Model file for the job. Use its own axes, mm. Face numbers are marked on the shaded views. Coordinates: 2 decimals unless noted, no trailing zeros. Order: outer loops, then holes, each group sorted by start corner. A loop starts at its lowest first (then second) coordinate and runs counter-clockwise, first axis right, second up. Notation, with made-up numbers: M 70,27 L 101,27 A25 ccw 101,58 Z; hole C -14,5.25 d4. An arc over 180 degrees is marked long. Return JSON: item names as keys, results as strings.
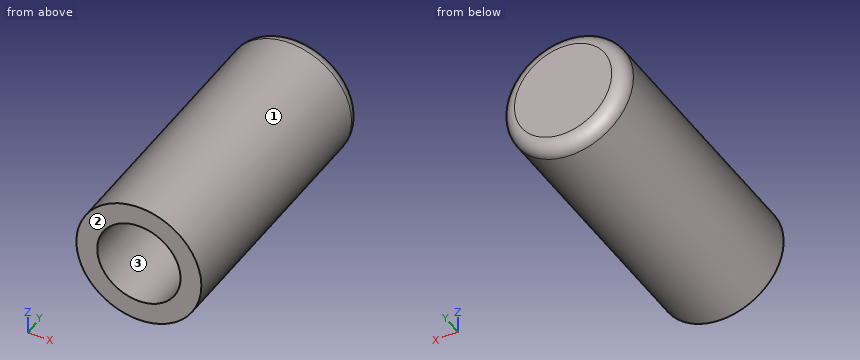
```python
from build123d import *

# Parameters (mm, degrees)
SKETCH2_R           = 4.5
SKETCH2_R_2         = 3
BOSS_EXTRUDE1_DEPTH = 20
SKETCH2_2_R         = 3
BOSS_EXTRUDE2_DEPTH = 2
FILLET1_R           = 1


with BuildPart() as part:
    # Sketch2 → Boss-Extrude1 (new body)
    with BuildSketch(Plane(origin=(0, 0, 0), x_dir=(1, 0, 0), z_dir=(0, 1, 0))):
        Circle(SKETCH2_R)
        Circle(SKETCH2_R_2, mode=Mode.SUBTRACT)
    extrude(amount=-BOSS_EXTRUDE1_DEPTH)

    # Sketch2<2> → Boss-Extrude2 (add)
    with BuildSketch(Plane(origin=(0, 0, 0), x_dir=(1, 0, 0), z_dir=(0, 1, 0))):
        Circle(SKETCH2_2_R)
    extrude(amount=-BOSS_EXTRUDE2_DEPTH)

    # Fillet1
    fillet1_edges = [part.edges().sort_by_distance(p)[0] for p in [
        (-4.5, 0, 0),
    ]]
    fillet(fillet1_edges, radius=FILLET1_R)


solid = part.part
```
Item 1: Saw through at C-C (z = 0). Write the cut outline in (x, y), and give its area (3 significant figures).
Check result:
{"outline": "M -4.5,-20 L -3,-20 L -3,-2 L 3,-2 L 3,-20 L 4.5,-20 L 4.5,-1 A1 ccw 3.5,0 L -3.5,0 A1 ccw -4.5,-1 Z", "area": "71.6 mm2"}
Item 2: Saw through at B-B (y = -5). Write the cut outline in (x, z).
Check result:
{"outline": "C 0,0 d9; hole C 0,0 d6"}
Item 3: Wall check: line 1 (Z direction, x = 0, y = -7); line 2 (Y direction, x = 2.5, z = 1). Give the ranges that are in metal, low to high.
Check result:
{"line 1": "z = -4.5 to -3, 3 to 4.5", "line 2": "y = -2 to 0"}
Item 4: Drop flat-ended pins along their axis: pin 1 Ø3 at (x, y) = (3, -11) entering from -Z; pin 2 Ø2 at (x, y) = (-2, -4) entering from -Z; pin 3 Ø5 at (y, z) = (-11.5, -0.5) entering from +X. Give the stop position or say it passes through.
Check result:
{"pin 1": "stops at z = -4.24", "pin 2": "stops at z = -4.39", "pin 3": "stops at x = 4.5"}
Item 5: Saw through at A-A (x = 0). Write the cut outline in (y, z), and give its area (3 significant figures).
Check result:
{"outline": "M -20,-4.5 L -1,-4.5 A1 ccw 0,-3.5 L 0,3.5 A1 ccw -1,4.5 L -20,4.5 L -20,3 L -2,3 L -2,-3 L -20,-3 Z", "area": "71.6 mm2"}
Item 6: Pull direction X, two halves, no side cores. Call the marked faces 1, 2 and 3: +X half, -X half, draft (parallel to the pull), parting line (faces both ways), or undercut.
Check result:
{"face 1": "parting line", "face 2": "draft", "face 3": "undercut"}
